```python
from build123d import *

# Parameters (mm, degrees)
SKETCH_W      = 38
SKETCH_H      = 50
PAD_DEPTH     = 19
SKETCH001_R   = 6
HOLE_DEPTH    = 38.001
SKETCH002_R   = 6
HOLE001_DEPTH = 38.001
CHAMFER_SIZE  = 1


with BuildPart() as part:
    # Sketch → Pad (new body, symmetric)
    with BuildSketch(Plane.YZ):
        Rectangle(SKETCH_W, SKETCH_H)
    extrude(amount=PAD_DEPTH, both=True)

    # Sketch001 (on Face6 of Pad) → Hole (cut, through all)
    with BuildSketch(Plane.YZ.offset(19)):
        with Locations((0, 6)):
            Circle(SKETCH001_R)
    extrude(amount=-HOLE_DEPTH, mode=Mode.SUBTRACT)

    # Sketch002 (on Face2 of Hole) → Hole001 (cut, through all)
    with BuildSketch(Plane(origin=(0, -19, 0), x_dir=(0, 0, -1), z_dir=(0, -1, 0))):
        with Locations((6, 0)):
            Circle(SKETCH002_R)
    extrude(amount=-HOLE001_DEPTH, mode=Mode.SUBTRACT)

    # Chamfer
    chamfer_edges = [part.edges().sort_by_distance(p)[0] for p in [
        (-19, 0, -25),
        (0, -19, -25),
        (19, 0, -25),
        (0, 19, -25),
        (-19, -19, 0),
        (0, -19, 25),
        (-19, 0, 25),
        (-19, 19, 0),
        (0, 19, 25),
        (19, 19, 0),
        (19, -19, 0),
        (19, 0, 25),
    ]]
    chamfer(chamfer_edges, length=CHAMFER_SIZE)


solid = part.part
```
Part model, mm, in its own coordinate system. Round coordinates to 2 decimals unless told otherwise and drop trailing zeros. Write each loop counter-clockwise with the first axis right and the second up, starting at its lowest first coordinate (ties: lowest second). Pieces come first, ordered by that corner, then holes. Notation, with made-up numbers: (-28.75, -12) -> (20.25, -12) arc R17 ccw to (20.25, 1) -> close; hole circle Ø5 at (-23, 33). An arc over 180 degrees is marked (long way). Return JSON: item names as keys, results as strings. Group by question number.
Q1. Probe L1, parallel to X at y = -5.5, z = -6; L2, parallel to Y at x = -17, z = 5; L3, parallel to Z at x = -8.5, y = 0. List the from-to ranges inside material, lowest first. Write a range as [from, to].
Q2. Saw through at C-C on y = 0. Write the cut outline in (x, z).
Q3. Saw through at A-A on x = 0. Write the cut outline in (y, z), plus the area to 3 significant figures.
Q4. Saw through at D-D on x = -16. Write the cut outline in (y, z).
Q5. Saw through at B-B on z = -6. Write the cut outline in (x, y), plus the area to 3 significant figures.
Q6. Mould opens along Z. For faces 1 (the flat face through (0, 0, 25)), 2 (the cylindrical face through (-3.65, -0.27, -1.24)), 3 (the flat face through (0, 0, -25)) say: pulls with the +Z half, pulls with the -Z half, needs draft (parallel to the pull), parting line crosses it, or undercut.
Q7. Pin check, flat tip, straight feed: pin 1 (9.5 mm diameter, centred on x = 0, z = -6, fed in from +Y). Stop position of the tip, or through.
Answer:
{
 "1": {"L1": "[-19, -6], [6, 19]", "L2": "[-19, -5.92], [5.92, 19]", "L3": "[-25, 0], [12, 25]"},
 "2": {"outline": "(-19, -24) -> (-18, -25) -> (18, -25) -> (19, -24) -> (19, 0) -> (-19, 0) -> close; (-19, 12) -> (19, 12) -> (19, 24) -> (18, 25) -> (-18, 25) -> (-19, 24) -> close; hole circle Ø12 at (0, -6)"},
 "3": {"outline": "(-19, -24) -> (-18, -25) -> (18, -25) -> (19, -24) -> (19, -12) -> (-19, -12) -> close; (-19, 0) -> (19, 0) -> (19, 24) -> (18, 25) -> (-18, 25) -> (-19, 24) -> close; hole circle Ø12 at (0, 6)", "area": "1,330 mm2"},
 "4": {"outline": "(-19, -24) -> (-18, -25) -> (18, -25) -> (19, -24) -> (19, 24) -> (18, 25) -> (-18, 25) -> (-19, 24) -> close; hole circle Ø12 at (0, 6)"},
 "5": {"outline": "(-19, -18) -> (-18, -19) -> (-6, -19) -> (-6, 19) -> (-18, 19) -> (-19, 18) -> close; (6, -19) -> (18, -19) -> (19, -18) -> (19, 18) -> (18, 19) -> (6, 19) -> close", "area": "986 mm2"},
 "6": {"face 1": "pulls with the +Z half", "face 2": "undercut", "face 3": "pulls with the -Z half"},
 "7": {"pin 1": "through"}
}
